For this review, take the finished solid that the model builds, in its own axes (mm). Face numbers are marked on the shaded views. A direction names the side the tool comes from. Coordinates: 2 decimals unless noted, no trailing zeros. Loops run counter-clockwise (first coordinate to the right, second up) from the corner with the lowest first, then second, coordinate; pieces in that order, holes last. Notation, with made-up numbers: (6, -3.5) - (37, -3.5) arc R14 cw to (37, 0.5) - close; hole circle Ø5 at (15.5, -31). An arc over 180 degrees is marked (long way). One line per item, written item: value. Start each with the question number.
1. For the marked faces 1 and 2, list the 3-axis set-ups (+Z, -Z, +X, -X, +Y, -Y) from which the entire face can be reached by the end or side of a thin tool; tool diameter is ignored.
2. Take a section at B-B, the plane x = -43. State the section outline as (y, z) points, and give its area (3 significant figures).
3. Take a section at D-D, the plane x = -38. State the section outline as (y, z) points.
4. Take a section at A-A, the plane z = -16. State the section outline as (x, y) points, and give its area (3 significant figures).
5. The part is to be moulded in two halves that separate along Z. For the marked faces 3, 4, 5 and 6, say which applies: released by +Z, released by -Z, zero draft, split by the parting line, or undercut.
6. Insertion check: pin 1 (3 mm diameter, centred on x = -17.5, y = -12.5, fed in from -Z); pin 2 (4 mm diameter, centred on x = -42, z = 0, fed in from -Y). Each pin has a flat end and moves straight along its axis. Give the tip position at first contact, or say it passes through.
7. Take a section at C-C, the plane y = 0. State the section outline as (x, z) points, and give its area (3 significant figures).
8. To check wall thickness, follow line 1 (Y direction, x = -2, z = 0); line 2 (Z direction, x = -15, y = 12.5); line 3 (X direction, y = 0, z = -23.8). State the ranges of each line that lie inside material, in increasing order. Write a range as from..to.
```python
from build123d import *

# Parameters (mm, degrees)
SKETCH1_W           = 50
SKETCH1_H           = 50
BOSS_EXTRUDE1_DEPTH = 50
SKETCH2_W           = 40
SKETCH2_H           = 40
CUT_EXTRUDE1_DEPTH  = 51
SKETCH4_R           = 15
CUT_EXTRUDE2_DEPTH  = 51


with BuildPart() as part:
    # Sketch1 → Boss-Extrude1 (new body)
    with BuildSketch(Plane(origin=(0, 0, 0), x_dir=(0, 0, -1), z_dir=(1, 0, 0))):
        Rectangle(SKETCH1_W, SKETCH1_H)
    extrude(amount=-BOSS_EXTRUDE1_DEPTH)

    # Sketch2 → Cut-Extrude1 (cut, through all)
    with BuildSketch(Plane(origin=(0, 25, 0), x_dir=(1, 0, 0), z_dir=(0, 1, 0))):
        with Locations((-25, 0)):
            Rectangle(SKETCH2_W, SKETCH2_H)
    extrude(amount=-CUT_EXTRUDE1_DEPTH, mode=Mode.SUBTRACT)

    # Sketch4 → Cut-Extrude2 (cut, through all)
    with BuildSketch(Plane(origin=(0, 0, 0), x_dir=(0, 0, -1), z_dir=(1, 0, 0))):
        Circle(SKETCH4_R)
    cut_extrude2 = extrude(amount=-CUT_EXTRUDE2_DEPTH, mode=Mode.SUBTRACT)

    # Mirror4: Cut-Extrude2 across plane
    add(cut_extrude2.mirror(Plane(origin=(-12.5, 0, -12.5), x_dir=(-0.707106781, 0, 0.707106781), z_dir=(0.707106781, 0, 0.707106781))), mode=Mode.SUBTRACT)


solid = part.part
```
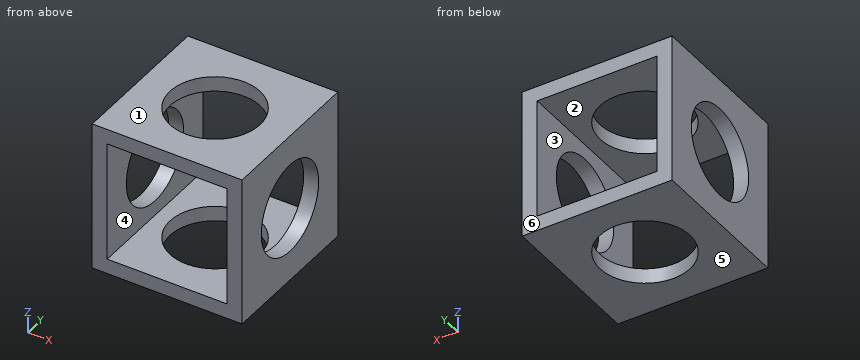
Solutions:
1. face 1: +Z, +X, -X, +Y, -Y
1. face 2: +Y, -Y
2. outline: (-25, -25) - (25, -25) - (25, -20) - (-25, -20) - close; (-25, 20) - (25, 20) - (25, 25) - (-25, 25) - close
2. area: 500 mm2
3. outline: (-25, -25) - (-7.48, -25) - (-7.48, -20) - (-25, -20) - close; (-25, 20) - (-7.48, 20) - (-7.48, 25) - (-25, 25) - close; (7.48, -25) - (25, -25) - (25, -20) - (7.48, -20) - close; (7.48, 20) - (25, 20) - (25, 25) - (7.48, 25) - close
4. outline: (-50, -25) - (-45, -25) - (-45, 25) - (-50, 25) - close; (-5, -25) - (0, -25) - (0, 25) - (-5, 25) - close
4. area: 500 mm2
5. face 3: undercut
5. face 4: undercut
5. face 5: released by -Z
5. face 6: zero draft
6. pin 1: z = -25
6. pin 2: through
7. outline: (-50, -25) - (-40, -25) - (-40, -20) - (-45, -20) - (-45, -15) - (-50, -15) - close; (-50, 15) - (-45, 15) - (-45, 20) - (-40, 20) - (-40, 25) - (-50, 25) - close; (-10, -25) - (0, -25) - (0, -15) - (-5, -15) - (-5, -20) - (-10, -20) - close; (-10, 20) - (-5, 20) - (-5, 15) - (0, 15) - (0, 25) - (-10, 25) - close
7. area: 300 mm2
8. line 1: -25..-15, 15..25
8. line 2: -25..-20, 20..25
8. line 3: -50..-40, -10..0
